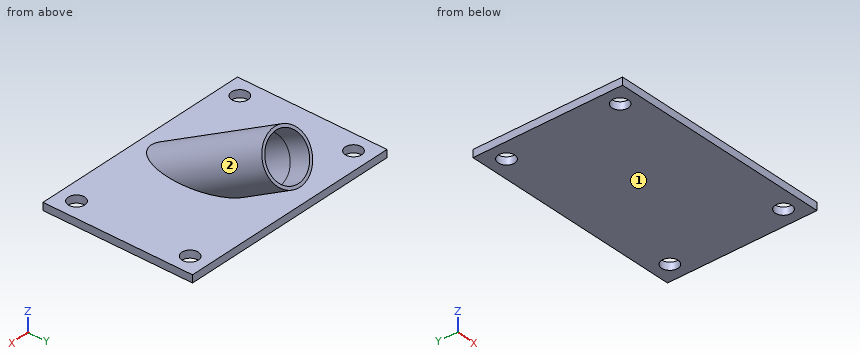
```python
from build123d import *

# Parameters (mm, degrees)
SZKIC1_W                                = 150
SZKIC1_H                                = 100
DODANIE_WYCI_GNI_CIE1_DEPTH             = 5
OTW_R_POD_RUB_M101_D                    = 11
LUSTRO1_AT_THE_SECOND_PLANE_COPY_1_D    = 11
SZKIC4_R                                = 17
SZKIC4_R_2                              = 15
DODANIE_WYCI_GNI_CIE2_DEPTH             = 15
DODANIE_WYCI_GNI_CIE2_DIRECTION_2_REACH = 91.103


with BuildPart() as part:
    # Szkic1 → Dodanie-wyciągnięcie1 (new body)
    with BuildSketch(Plane.XY):
        Rectangle(SZKIC1_W, SZKIC1_H)
    extrude(amount=DODANIE_WYCI_GNI_CIE1_DEPTH)

    # Otwór pod śrubę M101 (through all)
    with Locations(Plane.XY.offset(5)):
        with Locations((-63, 38)):
            otw_r_pod_rub_m101 = Hole(OTW_R_POD_RUB_M101_D / 2)

    # Lustro1: Otwór pod śrubę M101 across plane
    add(otw_r_pod_rub_m101.mirror(Plane.ZX), mode=Mode.SUBTRACT)

    # Lustro1 at the second plane: Otwór pod śrubę M101 across plane
    add(otw_r_pod_rub_m101.mirror(Plane(origin=(0, 0, 0), x_dir=(0, 0, 1), z_dir=(1, 0, 0))), mode=Mode.SUBTRACT)

    # Lustro1 at the second plane copy 1 (through all)
    with Locations(Plane(origin=(0, 0, 5), x_dir=(-1, 0, 0), z_dir=(0, 0, 1))):
        with Locations((-63, 38)):
            Hole(LUSTRO1_AT_THE_SECOND_PLANE_COPY_1_D / 2)

    # Szkic4 → Dodanie-wyciągnięcie2 (add)
    with BuildSketch(Plane(origin=(0, 39.665063509, 22.900635095), x_dir=(-1, 0, 0), z_dir=(0, 0.866025404, 0.5))):
        with Locations(Location((0, 8.683075721, 0), (0, 0, 90))):  # turned: the seam where the file's is
            Circle(SZKIC4_R)
        with Locations(Location((0, 8.683075721, 0), (0, 0, 90))):  # turned: the seam where the file's is
            Circle(SZKIC4_R_2, mode=Mode.SUBTRACT)
    extrude(amount=DODANIE_WYCI_GNI_CIE2_DEPTH)

    # Dodanie-wyciągnięcie2 direction 2: up to this face of the body (flat: up to its plane)
    dodanie_wyci_gni_cie2_direction_2_end = Plane(part.part.faces().sort_by_distance((0, 0, 5))[0])
    # Szkic4 → Dodanie-wyciągnięcie2 direction 2 (add, up to the picked face)
    with BuildSketch(Plane(origin=(0, 39.665063509, 22.900635095), x_dir=(-1, 0, 0), z_dir=(0, 0.866025404, 0.5)), mode=Mode.PRIVATE) as dodanie_wyci_gni_cie2_direction_2_sk1:
        with Locations(Location((0, 8.683075721, 0), (0, 0, 90))):  # turned: the seam where the file's is
            Circle(SZKIC4_R)
        with Locations(Location((0, 8.683075721, 0), (0, 0, 90))):  # turned: the seam where the file's is
            Circle(SZKIC4_R_2, mode=Mode.SUBTRACT)
    dodanie_wyci_gni_cie2_direction_2_tool1 = split(extrude(dodanie_wyci_gni_cie2_direction_2_sk1.sketch, amount=-DODANIE_WYCI_GNI_CIE2_DIRECTION_2_REACH, mode=Mode.PRIVATE), bisect_by=dodanie_wyci_gni_cie2_direction_2_end, keep=Keep.BOTH, mode=Mode.PRIVATE)
    add(dodanie_wyci_gni_cie2_direction_2_tool1.solids().sort_by(Axis((0, 43.583109, 16.114381), (0, -0.866025404, -0.5)))[0])


solid = part.part
```
Check sheet for the modelled part. Datum: model origin and axes. Units: mm. Face numbers are marked on the shaded views. Round coordinates to 2 decimals unless told otherwise and drop trailing zeros. Order: outer loops, then holes, each group sorted by start corner. A loop starts at its lowest first (then second) coordinate and runs counter-clockwise, first axis right, second up. Notation, with made-up numbers: (-23, -22.75) - (30, -22.75) arc R8 ccw to (30, -7.75) - close; hole circle Ø10 at (59.5, -24). An arc over 180 degrees is marked (long way). Answer as CSV lines item,"result". Start each with the question number.
1) Section check C-C (x = 5). Record the cut outline in (y, z).
2) Section check A-A (x = -63). Record the cut outline in (y, z).
3) Depth check by flat-ended pin: pin 1 (10 mm diameter, centred on x = -63, y = 38, fed in from +Z); pin 2 (12 mm diameter, centred on y = 33, z = 46, fed in from +X); pin 3 (3 mm diameter, centred on y = 22.5, z = 28.5, fed in from -X); pin 4 (3 mm diameter, centred on x = 29.5, y = -28.5, fed in from +Z). Enter the tip coordinate at first touch or a pass-through.
4) Scan lines: probe 1 along Y at (x, z) = (63, 3.05); probe 2 along Z at (x, y) = (6.5, 25); probe 3 along Z at (x, y) = (65.5, -4). Record each from-to range of solid material in increasing order.
5) Section check D-D (x = 43). Record the cut outline in (y, z), then the cut area to 3 significant figures.
6) Section check B-B (y = 38). Give the number of separate pieces and of enclosed holes in the cut face, then the cut area to 3 significant figures.
7) Draft check along Z on the marked faces 1 and 2. Enter one of: +Z half, -Z half, draft (parallel to the pull), parting line (faces both ways), or undercut.
Determined:
1,outline,"(-50, 0) - (50, 0) - (50, 5) - (23.79, 5) - (56.44, 23.85) - (55.38, 25.67) - (19.58, 5) - (-36.99, 5) - (41.24, 50.17) - (40.19, 51.99) - (-41.2, 5) - (-50, 5) - close"
2,outline,"(-50, 0) - (-43.5, 0) - (-43.5, 5) - (-50, 5) - close; (-32.5, 0) - (32.5, 0) - (32.5, 5) - (-32.5, 5) - close; (43.5, 0) - (50, 0) - (50, 5) - (43.5, 5) - close"
3,pin 1,"through"
3,pin 2,"x = 14.63"
3,pin 3,"x = -16.69"
3,pin 4,"z = 5"
4,probe 1,"-50 to -43.5, -32.5 to 32.5, 43.5 to 50"
4,probe 2,"0 to 5, 6.32 to 8.85, 40.07 to 42.6"
4,probe 3,"0 to 5"
5,outline,"(-50, 0) - (50, 0) - (50, 5) - (-50, 5) - close"
5,area,"500 mm^2"
6,separate pieces,"4"
6,enclosed holes,"1"
6,area,"872 mm^2"
7,face 1,"-Z half"
7,face 2,"undercut"
